Geometry: final body of the model. Coordinates: model frame, mm. Give positions to 0.01 mm unless a question says otherwise; leave off trailing zeros. Use one line per item in the form item = value.
```python
from build123d import *

# Parameters (mm, degrees)
ACRYLIC_2MM_START        = -12
ACRYLIC_2MM_DEPTH        = 2
HINGE_CLEARANCE_0_START  = -9.8
HINGE_CLEARANCE_0_DEPTH  = 2.4
HINGE_CLEARANCE_1_START  = -9.8
HINGE_CLEARANCE_1_DEPTH  = 2.4
M3_CLEARANCE_0_START     = -9.8
M3_CLEARANCE_0_PROFILE_R = 1.7
M3_CLEARANCE_0_DEPTH     = 2.4
M3_CLEARANCE_1_START     = -9.8
M3_CLEARANCE_1_PROFILE_R = 1.7
M3_CLEARANCE_1_DEPTH     = 2.4
M3_CLEARANCE_2_START     = -9.8
M3_CLEARANCE_2_PROFILE_R = 1.7
M3_CLEARANCE_2_DEPTH     = 2.4
M3_CLEARANCE_3_START     = -9.8
M3_CLEARANCE_3_PROFILE_R = 1.7
M3_CLEARANCE_3_DEPTH     = 2.4
KEYS_ACCESS_R1_5_START   = -9.8
KEYS_ACCESS_R1_5_DEPTH   = 2.4


with BuildPart() as part:
    # Acrylic_2mm_profile → Acrylic_2mm (new body)
    with BuildSketch(Plane.XY.offset(ACRYLIC_2MM_START)):
        with BuildLine():
            Line((0, -7), (190, -7))
            ThreePointArc((190, -7), (192.121320344, -6.121320344), (193, -4))
            Line((193, -4), (193, 160))
            ThreePointArc((193, 160), (192.121320344, 162.121320344), (190, 163))
            Line((190, 163), (0, 163))
            ThreePointArc((0, 163), (-2.121320344, 162.121320344), (-3, 160))
            Line((-3, 160), (-3, -4))
            ThreePointArc((-3, -4), (-2.121320344, -6.121320344), (0, -7))
        make_face()
    extrude(amount=ACRYLIC_2MM_DEPTH)

    # Hinge_clearance_0_profile → Hinge_clearance_0 (cut)
    with BuildSketch(Plane.XY.offset(HINGE_CLEARANCE_0_START)):
        with BuildLine():
            Line((-4, 113.5), (8.8, 113.5))
            ThreePointArc((8.8, 113.5), (10.214213562, 114.085786438), (10.8, 115.5))
            Line((10.8, 115.5), (10.8, 130.5))
            ThreePointArc((10.8, 130.5), (10.214213562, 131.914213562), (8.8, 132.5))
            Line((8.8, 132.5), (-4, 132.5))
            ThreePointArc((-4, 132.5), (-5.414213562, 131.914213562), (-6, 130.5))
            Line((-6, 130.5), (-6, 115.5))
            ThreePointArc((-6, 115.5), (-5.414213562, 114.085786438), (-4, 113.5))
        make_face()
    extrude(amount=-HINGE_CLEARANCE_0_DEPTH, mode=Mode.SUBTRACT)

    # Hinge_clearance_1_profile → Hinge_clearance_1 (cut)
    with BuildSketch(Plane.XY.offset(HINGE_CLEARANCE_1_START)):
        with BuildLine():
            Line((181.2, 113.5), (194, 113.5))
            ThreePointArc((194, 113.5), (195.414213562, 114.085786438), (196, 115.5))
            Line((196, 115.5), (196, 130.5))
            ThreePointArc((196, 130.5), (195.414213562, 131.914213562), (194, 132.5))
            Line((194, 132.5), (181.2, 132.5))
            ThreePointArc((181.2, 132.5), (179.785786438, 131.914213562), (179.2, 130.5))
            Line((179.2, 130.5), (179.2, 115.5))
            ThreePointArc((179.2, 115.5), (179.785786438, 114.085786438), (181.2, 113.5))
        make_face()
    extrude(amount=-HINGE_CLEARANCE_1_DEPTH, mode=Mode.SUBTRACT)

    # M3_clearance_0_profile → M3_clearance_0 (cut)
    with BuildSketch(Plane.XY.offset(M3_CLEARANCE_0_START)):
        with Locations((5, 5)):
            Circle(M3_CLEARANCE_0_PROFILE_R)
    extrude(amount=-M3_CLEARANCE_0_DEPTH, mode=Mode.SUBTRACT)

    # M3_clearance_1_profile → M3_clearance_1 (cut)
    with BuildSketch(Plane.XY.offset(M3_CLEARANCE_1_START)):
        with Locations((185, 5)):
            Circle(M3_CLEARANCE_1_PROFILE_R)
    extrude(amount=-M3_CLEARANCE_1_DEPTH, mode=Mode.SUBTRACT)

    # M3_clearance_2_profile → M3_clearance_2 (cut)
    with BuildSketch(Plane.XY.offset(M3_CLEARANCE_2_START)):
        with Locations((5, 155)):
            Circle(M3_CLEARANCE_2_PROFILE_R)
    extrude(amount=-M3_CLEARANCE_2_DEPTH, mode=Mode.SUBTRACT)

    # M3_clearance_3_profile → M3_clearance_3 (cut)
    with BuildSketch(Plane.XY.offset(M3_CLEARANCE_3_START)):
        with Locations((185, 155)):
            Circle(M3_CLEARANCE_3_PROFILE_R)
    extrude(amount=-M3_CLEARANCE_3_DEPTH, mode=Mode.SUBTRACT)

    # Keys_access_R1_5_profile → Keys_access_R1_5 (cut)
    with BuildSketch(Plane.XY.offset(KEYS_ACCESS_R1_5_START)):
        with BuildLine():
            Line((112.12500058, 81.24999704), (130.9999982, 81.24999704))
            ThreePointArc((130.9999982, 81.24999704), (132.060658372, 81.689336868), (132.4999982, 82.74999704))
            Line((132.4999982, 82.74999704), (132.4999982, 85.74999974))
            ThreePointArc((132.4999982, 85.74999974), (132.060658372, 86.810659912), (130.9999982, 87.24999974))
            Line((130.9999982, 87.24999974), (112.12500058, 87.24999974))
            ThreePointArc((112.12500058, 87.24999974), (111.064340408, 86.810659912), (110.62500058, 85.74999974))
            Line((110.62500058, 85.74999974), (110.62500058, 82.74999704))
            ThreePointArc((110.62500058, 82.74999704), (111.064340408, 81.689336868), (112.12500058, 81.24999704))
        make_face()
    extrude(amount=-KEYS_ACCESS_R1_5_DEPTH, mode=Mode.SUBTRACT)


solid = part.part
```
(1) Material intervals for L1, parallel to Y at x = 5, z = -10.8; L2, parallel to X at y = 155, z = -10.6; L3, parallel to X at y = 85, z = -10.65 (3 decimals), sorted ascending. Write a range as from..to.
Solution:
L1 = -7..3.3, 6.7..113.5, 132.5..153.3, 156.7..163
L2 = -3..3.3, 6.7..183.3, 186.7..193
L3 = -3..110.625, 132.5..193
(2) Cut plane A-A (z = -10.95). Give the number of separate pieces and of enclosed holes in the cut face, plus the area to 3 significant figures.
Solution:
separate_pieces = 1
enclosed_holes = 5
area = 32,600 mm2
(3) Pin query (flat end, axial travel): P1, Ø1, axis at y = 123, z = -11.5, coming from the -X side; P2, Ø1, axis at y = 126.5, z = -10.5, coming from the +X side; P3, Ø2, axis at x = 185, y = 5, coming from the -Z side. Return the tip coordinate at first contact, or that it passes through.
Solution:
P1 = 10.8
P2 = 179.2
P3 = through
